Work out the finished part from the listing and answer in its coordinate system (mm). A direction names the side the tool comes from. Give positions to 0.01 mm unless a question says otherwise; leave off trailing zeros. Loops run counter-clockwise (first coordinate to the right, second up) from the corner with the lowest first, then second, coordinate; pieces in that order, holes last.
```python
from build123d import *

# Parameters (mm, degrees)
SK_BASE_W                  = 92.82
SK_BASE_H                  = 31
BASE_PLATE_DEPTH           = 4
SK_BLOCK_W                 = 42
SK_BLOCK_H                 = 29
CAMERA_BLOCK_DEPTH         = 5
SK_PINHOLE_R               = 1.8
SLIDE_PIN_HOLE_DEPTH       = 4
CABLE_TIE_SLOTS_DEPTH      = 95.534662426
CABLE_TIE_SLOTS_DEPTH_BACK = 95.534662426
SK_TIESLOTS_W              = 2
SK_TIESLOTS_H              = 8


with BuildPart() as part:
    # Sk_Base → Base Plate (new body)
    with BuildSketch(Plane(origin=(0, 0, 0), x_dir=(1, 0, 0), z_dir=(0, 1, 0))):
        with Locations((46.41, 0)):
            Rectangle(SK_BASE_W, SK_BASE_H)
    extrude(amount=BASE_PLATE_DEPTH)

    # Sk_Block → Camera Block (add)
    with BuildSketch(Plane(origin=(0, 4, 0), x_dir=(1, 0, 0), z_dir=(0, 1, 0))):
        with Locations((46.41, 0)):
            Rectangle(SK_BLOCK_W, SK_BLOCK_H)
    extrude(amount=CAMERA_BLOCK_DEPTH)

    # Sk_PinHole → Slide Pin Hole (cut)
    with BuildSketch(Plane(origin=(0, 0, 0), x_dir=(1, 0, 0), z_dir=(0, 1, 0))):
        with Locations(Location((46.41, 0, 0), (0, 0, 270))):
            Circle(SK_PINHOLE_R)
    extrude(amount=SLIDE_PIN_HOLE_DEPTH, mode=Mode.SUBTRACT)

    # Sk_TieSlots → Cable Tie Slots (cut, two sides: drawn at the far end of the back side and taken through both)
    with BuildSketch(Plane(origin=(0, 0, 0), x_dir=(1, 0, 0), z_dir=(0, 1, 0)).offset(-CABLE_TIE_SLOTS_DEPTH_BACK)):
        with Locations((5, 0)):
            Rectangle(SK_TIESLOTS_W, SK_TIESLOTS_H)
        with Locations((23, 0)):
            Rectangle(SK_TIESLOTS_W, SK_TIESLOTS_H)
    extrude(amount=CABLE_TIE_SLOTS_DEPTH + CABLE_TIE_SLOTS_DEPTH_BACK, mode=Mode.SUBTRACT)


solid = part.part
```
Q1. Given pin 1 (4 mm diameter, centred on x = 48.5, y = 6.5, fed in from +Z); pin 2 (1.5 mm diameter, centred on y = 6.5, z = -5.5, fed in from +X); pin 3 (1.5 mm diameter, centred on x = 40.5, y = 7, fed in from -Z), each flat-ended and moving along its own axis, determine where each tip first touches the part or whether it passes through.
Q2. Section A-A on z = 0 is taken. Give the vertices of the cut face in (x, y), plus the area to 3 significant figures.
Q3. Section D-D on y = 7.5 is taken. Give the vertices of the cut face in (x, z).
Q4. Which of the six approach directions +Z, -Z, +X, -X, +Y, -Y give full straight-line access (tool end or side, diameter ignored) to faces 1 (the face through (46, 6, -14.5)), 2 (the face through (25.41, 6, 0)), 3 (the face through (48.2, 2, -0.2)), 4 (the face through (5, 2, -4))?
Q5. Determine the mould class of faces 5 (the face through (46, 2, -15.5)), 6 (the face through (4, 2, 0)), 7 (the face through (0, 2, 0)), 8 (the face through (5, 2, 4)) for opening direction Z: +Z half, -Z half, draft (parallel to the pull), parting line (faces both ways), or undercut.
Q6. Consider line 1 along X through (y, z) = (2.5, 0); line 2 along Y through (x, z) = (81, -3.5); line 3 along X through (y, z) = (5.75, 7.5). Determine where each line is inside the solid, lowest interval first.
Q7. Section C-C on z = -5.5 is taken. Give the vertices of the cut face in (x, y).
Q8. Section B-B on x = 46.41 is taken. Give the vertices of the cut face in (y, z).
Check result:
1. pin 1: stops at z = 14.5
1. pin 2: stops at x = 67.41
1. pin 3: stops at z = -14.5
2. outline: (0, 0) - (4, 0) - (4, 4) - (0, 4) - close; (6, 0) - (22, 0) - (22, 4) - (6, 4) - close; (24, 0) - (44.61, 0) - (44.61, 4) - (48.21, 4) - (48.21, 0) - (92.82, 0) - (92.82, 4) - (67.41, 4) - (67.41, 9) - (25.41, 9) - (25.41, 4) - (24, 4) - close
2. area: 551 mm2
3. outline: (25.41, -14.5) - (67.41, -14.5) - (67.41, 14.5) - (25.41, 14.5) - close
4. face 1: -Z, +X, -X, +Y
4. face 2: +Z, -Z, -X, +Y
4. face 3: -Y
4. face 4: +Y, -Y
5. face 5: -Z half
5. face 6: undercut
5. face 7: draft
5. face 8: undercut
6. line 1: x = 0 to 4, 6 to 22, 24 to 44.61, 48.21 to 92.82
6. line 2: y = 0 to 4
6. line 3: x = 25.41 to 67.41
7. outline: (0, 0) - (92.82, 0) - (92.82, 4) - (67.41, 4) - (67.41, 9) - (25.41, 9) - (25.41, 4) - (0, 4) - close
8. outline: (0, -15.5) - (4, -15.5) - (4, -14.5) - (9, -14.5) - (9, 14.5) - (4, 14.5) - (4, 15.5) - (0, 15.5) - (0, 1.8) - (4, 1.8) - (4, -1.8) - (0, -1.8) - close
